Geometry: final body of the model. Coordinates: model frame, mm. A direction names the side the tool comes from. Give positions to 0.01 mm unless a question says otherwise; leave off trailing zeros. Loops run counter-clockwise (first coordinate to the right, second up) from the corner with the lowest first, then second, coordinate; pieces in that order, holes last. Notation, with made-up numbers: (-1, -3) -> (29, -3) arc R16 cw to (29, 22) -> close; hole circle Ø2 at (-22, 18). An arc over 180 degrees is marked (long way). Answer in a Markdown table with one row per item. Add a question column.
1) Section query A-A (y = 74.5). Return the cut outline in (x, z).
2) Section query D-D (y = 61.5). Return the cut outline in (x, z).
3) Access query for faces 1 (the conical face through (-11.947, 81.536, -9.959)), 2 (the flat face through (7, 70, -8)). Directions: +Z, -Z, +X, -X, +Y, -Y. A direction counts if a zero-diameter tool reaches every point of the face in a straight line with its end or side. Return the directions, or none.
4) Line query: line 1 (Y direction, x = 7.5, z = 12.5); line 2 (X direction, y = 50, z = 4.5); line 3 (Z direction, x = 12, y = 74) (3 decimals). Output: solid intervals per line, ascending. Write a range as from..to.
5) First-contact query: P1, Ø1.5, axis at y = 27.5, z = -0.5, coming from the +X side; P2, Ø4, axis at x = 8, y = 33.5, coming from the -Z side; P3, Ø2, axis at y = 35.5, z = 5, coming from the -X side. Flat tips, straight axial feed; report the tip coordinate or a pass-through.
6) Section query B-B (x = 0). Return the cut outline in (y, z).
7) Section query C-C (z = 0). Return the cut outline in (x, y).
```python
from build123d import *

# Parameters (mm, degrees)
SKETCH1_W           = 10
SKETCH1_H           = 70
BOSS_EXTRUDE1_DEPTH = 12
SKETCH3_OUTSIDE_W   = 60.55
SKETCH3_OUTSIDE_H   = 62.214
SKETCH3_OUTSIDE_R   = 15
CUT_EXTRUDE1_DEPTH  = 3
CUT_EXTRUDE1_DRAFT  = -50
CHAMFER1_SIZE       = 1


with BuildPart() as part:
    # Sketch1 → Revolve1 (revolve)
    with BuildSketch(Plane.XY, mode=Mode.PRIVATE) as revolve1_sk:
        with Locations((5, 35)):
            Rectangle(SKETCH1_W, SKETCH1_H)
    revolve(revolve1_sk.sketch.rotate(Axis((0, 70, 0), (0, -1, 0)), 180), axis=Axis((0, 70, 0), (0, -1, 0)))

    # Sketch2 → Boss-Extrude1 (add)
    with BuildSketch(Plane(origin=(0, 70, 0), x_dir=(1, 0, 0), z_dir=(0, 1, 0))):
        Polygon((13.331465099, -11.057668756), (16.241954599, 6.016553068), (2.9104895, 17.074221823), (-13.331465099, 11.057668756), (-16.241954599, -6.016553068), (-2.9104895, -17.074221823), align=None)
    extrude(amount=BOSS_EXTRUDE1_DEPTH)


with BuildPart() as cut_extrude1_tool:
    # Sketch3 outside → Cut-Extrude1 (with draft: the straight prism first)
    with BuildSketch(Plane(origin=(0, 82, 0), x_dir=(1, 0, 0), z_dir=(0, 1, 0))):
        Rectangle(SKETCH3_OUTSIDE_W, SKETCH3_OUTSIDE_H)
        Circle(SKETCH3_OUTSIDE_R, mode=Mode.SUBTRACT)
    extrude(amount=-CUT_EXTRUDE1_DEPTH)
    # Cut-Extrude1: the draft: its side faces are tilted about the plane it starts from
    cut_extrude1_sides = [cut_extrude1_tool.faces().sort_by_distance(p)[0] for p in [
        (0, 80.5, 31.107),
        (30.275, 80.5, 0),
        (0, 80.5, -31.107),
        (-30.275, 80.5, 0),
        (-15, 80.5, 0),
    ]]
    draft(cut_extrude1_sides, Plane(origin=(0, 82, 0), x_dir=(1, 0, 0), z_dir=(0, 1, 0)), CUT_EXTRUDE1_DRAFT)


with BuildPart() as part_1:
    add(part.part)

    # Cut-Extrude1: cut by cut_extrude1_tool
    add(cut_extrude1_tool.part, mode=Mode.SUBTRACT)

    # Chamfer1
    chamfer1_edges = [part_1.edges().sort_by_distance(p)[0] for p in [
        (10, 0, 0),
    ]]
    chamfer(chamfer1_edges, length=CHAMFER1_SIZE)


solid = part_1.part
```
Evaluation:
| question | item | result |
|---|---|---|
| 1 | outline | (-16.24, 6.02) -> (-13.33, -11.06) -> (2.91, -17.07) -> (16.24, -6.02) -> (13.33, 11.06) -> (-2.91, 17.07) -> close |
| 2 | outline | circle Ø20 at (0, 0) |
| 3 | face 1 | -Z, -X, +Y |
| 3 | face 2 | -Y |
| 4 | line 1 | 70..82 |
| 4 | line 2 | -8.93..8.93 |
| 4 | line 3 | -9.535..11.551 |
| 5 | P1 | x = 10 |
| 5 | P2 | z = -8 |
| 5 | P3 | x = -9.17 |
| 6 | outline | (0, -9) -> (1, -10) -> (70, -10) -> (70, -16) -> (81.16, -16) -> (82, -15) -> (82, 15) -> (81.16, 16) -> (70, 16) -> (70, 10) -> (1, 10) -> (0, 9) -> close |
| 7 | outline | (-15.22, 70) -> (-10, 70) -> (-10, 1) -> (-9, 0) -> (9, 0) -> (10, 1) -> (10, 70) -> (15.22, 70) -> (15.22, 81.82) -> (15, 82) -> (-15, 82) -> (-15.22, 81.82) -> close |
